Work out the finished part from the listing and answer in its coordinate system (mm). Face numbers are marked on the shaded views. Give positions to 0.01 mm unless a question says otherwise; leave off trailing zeros. Loops run counter-clockwise (first coordinate to the right, second up) from the corner with the lowest first, then second, coordinate; pieces in that order, holes last. Notation, with made-up numbers: (31.25, -39.75) -> (63.25, -39.75) arc R27 cw to (63.25, -13.75) -> close; hole circle Ø6 at (-24.5, -37). An arc over 180 degrees is marked (long way). Answer as CSV lines item,"result". Start each with the question number.
1. Find section A-A, the plane x = -26. Give the vertices of the cut face in (y, z) (3 decimals).
2. Determine the mould class of the marked faces 1 and 2 for opening direction Z: +Z half, -Z half, draft (parallel to the pull), parting line (faces both ways), or undercut.
3. Find section C-C, the plane z = 2.3. Give the vertices of the cut face in (x, y) (3 decimals), and give its area (3 significant figures).
4. Find the intervals of material crossed by line 1 along X through (y, z) = (-22, 2.8) (3 decimals); line 2 along Y through (x, z) = (27, 0.25) (3 decimals), in increasing order.
5. Find section B-B, the plane y = 25. Give the vertices of the cut face in (x, z) (3 decimals).
from build123d import *

# Parameters (mm, degrees)
SKETCH1_W           = 100
SKETCH1_H           = 80
BOSS_EXTRUDE1_DEPTH = 3.175
SKETCH4_W           = 100.51
SKETCH4_H           = 80.51
SKETCH4_W_2         = 87.47
SKETCH4_H_2         = 67.47
CUT_EXTRUDE3_DEPTH  = 10
SKETCH5_R           = 1.415
CUT_EXTRUDE4_DEPTH  = 10
SKETCH2_W           = 21.13
SKETCH2_H           = 65.13
CUT_EXTRUDE5_DEPTH  = 10
BOSS_EXTRUDE2_DEPTH = 3.175


with BuildPart() as part:
    # Sketch1 → Boss-Extrude1 (new body)
    with BuildSketch(Plane.XY):
        Rectangle(SKETCH1_W, SKETCH1_H)
    extrude(amount=BOSS_EXTRUDE1_DEPTH)

    # Sketch4 → Cut-Extrude3 (cut)
    with BuildSketch(Plane.XY.offset(3.175)):
        Rectangle(SKETCH4_W, SKETCH4_H)
        Rectangle(SKETCH4_W_2, SKETCH4_H_2, mode=Mode.SUBTRACT)
    extrude(amount=-CUT_EXTRUDE3_DEPTH, mode=Mode.SUBTRACT)

    # Sketch5 → Cut-Extrude4 (cut)
    with BuildSketch(Plane.XY.offset(3.175)):
        with Locations((-40.553019485, 30.553019485)):
            Circle(SKETCH5_R)
        with Locations((-40.553019485, -30.553019485)):
            Circle(SKETCH5_R)
        with Locations((40.553019485, -30.553019485)):
            Circle(SKETCH5_R)
        with Locations((40.553019485, 30.553019485)):
            Circle(SKETCH5_R)
    extrude(amount=-CUT_EXTRUDE4_DEPTH, mode=Mode.SUBTRACT)

    # Sketch2 → Cut-Extrude5 (cut)
    with BuildSketch(Plane.XY.offset(3.175)):
        with Locations((-25.65, 0)):
            Rectangle(SKETCH2_W, SKETCH2_H)
        with Locations((25.65, 0)):
            Rectangle(SKETCH2_W, SKETCH2_H)
    extrude(amount=-CUT_EXTRUDE5_DEPTH, mode=Mode.SUBTRACT)

    # Sketch6 → Boss-Extrude2 (add)
    with BuildSketch(Plane.XY.offset(3.175)):
        Polygon((-25.65, -32.565), (-15.085, -32.565), (-15.085, -27.475), (-25.65, -27.475), (-36.215, -27.475), (-36.215, -32.565), align=None)
        Polygon((25.65, -32.565), (36.215, -32.565), (36.215, -27.475), (25.65, -27.475), (15.085, -27.475), (15.085, -32.565), align=None)
        Polygon((15.085, 27.475), (15.085, 32.565), (25.65, 32.565), (36.215, 32.565), (36.215, 27.475), (25.65, 27.475), align=None)
        Polygon((-36.215, 27.475), (-36.215, 32.565), (-25.65, 32.565), (-15.085, 32.565), (-15.085, 27.475), (-25.65, 27.475), align=None)
    extrude(amount=-BOSS_EXTRUDE2_DEPTH)


solid = part.part
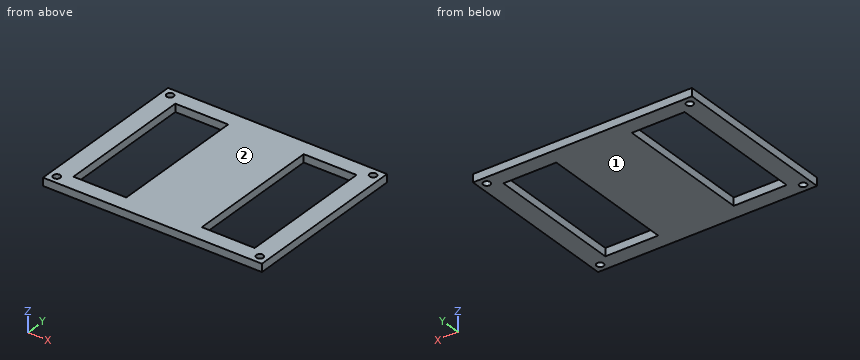
Resolved:
1,outline,"(-33.735, 0) -> (-27.475, 0) -> (-27.475, 3.175) -> (-33.735, 3.175) -> close; (27.475, 0) -> (33.735, 0) -> (33.735, 3.175) -> (27.475, 3.175) -> close"
2,face 1,"-Z half"
2,face 2,"+Z half"
3,outline,"(-43.735, -33.735) -> (43.735, -33.735) -> (43.735, 33.735) -> (-43.735, 33.735) -> close; hole circle Ø2.83 at (-40.553, -30.553); hole circle Ø2.83 at (-40.553, 30.553); hole (-36.215, -27.475) -> (-15.085, -27.475) -> (-15.085, 27.475) -> (-36.215, 27.475) -> close; hole (15.085, -27.475) -> (36.215, -27.475) -> (36.215, 27.475) -> (15.085, 27.475) -> close; hole circle Ø2.83 at (40.553, -30.553); hole circle Ø2.83 at (40.553, 30.553)"
3,area,"3,550 mm^2"
4,line 1,"x = -43.735 to -36.215, -15.085 to 15.085, 36.215 to 43.735"
4,line 2,"y = -33.735 to -27.475, 27.475 to 33.735"
5,outline,"(-43.735, 0) -> (-36.215, 0) -> (-36.215, 3.175) -> (-43.735, 3.175) -> close; (-15.085, 0) -> (15.085, 0) -> (15.085, 3.175) -> (-15.085, 3.175) -> close; (36.215, 0) -> (43.735, 0) -> (43.735, 3.175) -> (36.215, 3.175) -> close"
